```python
from build123d import *

# Parameters (mm, degrees)
SKETCH1_W           = 7
SKETCH1_H           = 7
BOSS_EXTRUDE1_DEPTH = 3
CUT_EXTRUDE1_DEPTH  = 7
CUT_EXTRUDE2_DEPTH  = 11
SKETCH4_R           = 1.8
CUT_EXTRUDE3_DEPTH  = 0.8
CUT_EXTRUDE4_DEPTH  = 0.4


with BuildPart() as part:
    # Sketch1 → Boss-Extrude1 (new body)
    with BuildSketch(Plane(origin=(0, 0, 0), x_dir=(1, 0, 0), z_dir=(0, 1, 0))):
        with Locations((3.5, 3.5)):
            Rectangle(SKETCH1_W, SKETCH1_H)
    extrude(amount=BOSS_EXTRUDE1_DEPTH)

    # Sketch2 → Cut-Extrude1 (cut)
    with BuildSketch(Plane.XY):
        Polygon((0, 0), (0.7, 3), (0, 3), align=None)
        Polygon((7, 0), (6.3, 3), (7, 3), align=None)
    extrude(amount=-CUT_EXTRUDE1_DEPTH, mode=Mode.SUBTRACT)

    # Sketch3 → Cut-Extrude2 (cut)
    with BuildSketch(Plane(origin=(0, 0, 0), x_dir=(0, 0, -1), z_dir=(1, 0, 0))):
        Polygon((0, 0), (0.7, 3), (0, 3), align=None)
        Polygon((7, 3), (6.3, 3), (7, 0), align=None)
    extrude(amount=CUT_EXTRUDE2_DEPTH, mode=Mode.SUBTRACT)

    # Sketch4 → Cut-Extrude3 (cut)
    with BuildSketch(Plane.XZ):
        with Locations(Location((3.5, -3.5, 0), (0, 0, 270))):
            Circle(SKETCH4_R)
    extrude(amount=-CUT_EXTRUDE3_DEPTH, mode=Mode.SUBTRACT)

    # Sketch5 → Cut-Extrude4 (cut)
    with BuildSketch(Plane(origin=(0, 3, 0), x_dir=(1, 0, 0), z_dir=(0, 1, 0))):
        with BuildLine():
            add(Edge.make_bspline(
                [(1.821714103, 3.488248698), (1.821961784, 3.531500253), (1.822448196, 3.616440725), (1.830876604, 3.741051587), (1.841985901, 3.86049575), (1.860077374, 3.974303397), (1.881359551, 4.083007187), (1.907977906, 4.186574853), (1.940043598, 4.284643186), (1.96555211, 4.347258757), (1.978064263, 4.377972255)],
                knots=[0, 0, 0, 0, 1.141009212, 2.240794809, 3.294380675, 4.305229195, 5.280013876, 6.216333343, 7.125095522, 8, 8, 8, 8], degree=3))
            add(Edge.make_bspline(
                [(1.978064263, 4.377972255), (1.998516886, 4.421635051), (2.039181575, 4.508447097), (2.114702293, 4.631119496), (2.200300575, 4.746809508), (2.295271713, 4.854910638), (2.397191064, 4.953795484), (2.506539435, 5.038426674), (2.619432008, 5.111662383), (2.699724257, 5.148495592), (2.739482532, 5.166734275)],
                knots=[0, 0, 0, 0, 1.031372299, 2.050613973, 3.077158538, 4.108712802, 5.127684358, 6.111366908, 7.06480644, 8, 8, 8, 8], degree=3))
            add(Edge.make_bspline(
                [(2.739482532, 5.166734275), (2.766470301, 5.177804055), (2.821019461, 5.200178904), (2.905795278, 5.228103887), (2.993787729, 5.250791674), (3.084360371, 5.271071912), (3.178392588, 5.285055803), (3.27512456, 5.296780816), (3.375085669, 5.302926099), (3.442700631, 5.303740345), (3.47706266, 5.304154146)],
                knots=[0, 0, 0, 0, 0.92659354, 1.872881803, 2.832850937, 3.813025581, 4.820167273, 5.851730198, 6.908245912, 8, 8, 8, 8], degree=3))
            add(Edge.make_bspline(
                [(3.47706266, 5.304154146), (3.538590536, 5.302611845), (3.659001433, 5.299593539), (3.834887941, 5.277792675), (4.001329981, 5.240979909), (4.157764144, 5.187771817), (4.305539157, 5.121260548), (4.443506895, 5.038760892), (4.571871554, 4.941165749), (4.690385205, 4.829813461), (4.797115236, 4.704898086), (4.890068226, 4.567586522), (4.968043218, 4.418522223), (5.032260126, 4.258116463), (5.081605981, 4.085845307), (5.117258315, 3.902194835), (5.138438688, 3.707029775), (5.140941529, 3.573137898), (5.142226923, 3.504374499)],
                knots=[0, 0, 0, 0, 1.064641025, 2.083517118, 3.061799897, 4.009540929, 4.938075217, 5.861300345, 6.78508344, 7.723570974, 8.670267188, 9.622657076, 10.586935816, 11.576069104, 12.607749008, 13.683335114, 14.81022093, 16, 16, 16, 16], degree=3))
            add(Edge.make_bspline(
                [(5.142226923, 3.504374499), (5.140971218, 3.436071549), (5.138526593, 3.303098467), (5.116950876, 3.109464875), (5.082776635, 2.92715322), (5.032236807, 2.75657997), (4.969936504, 2.596443536), (4.89115913, 2.448651271), (4.800152856, 2.311242808), (4.693574415, 2.187673494), (4.577055417, 2.075682155), (4.448853581, 1.979227653), (4.31189018, 1.896616215), (4.164920865, 1.829912739), (4.008903554, 1.777800449), (3.843329096, 1.740704804), (3.668112571, 1.718987832), (3.548170832, 1.715958568), (3.486878366, 1.714410557)],
                knots=[0, 0, 0, 0, 1.18845052, 2.313691126, 3.386664782, 4.412527756, 5.405809582, 6.372003093, 7.321919452, 8.268293321, 9.206237639, 10.129603466, 11.054616372, 11.9847576, 12.932764752, 13.912672021, 14.933336461, 16, 16, 16, 16], degree=3))
            add(Edge.make_bspline(
                [(3.486878366, 1.714410557), (3.424885779, 1.71596214), (3.303548476, 1.718999034), (3.126463104, 1.7406499), (2.959245037, 1.777757756), (2.802013351, 1.830053351), (2.653695695, 1.895743521), (2.51566143, 1.97751079), (2.387834254, 2.074576155), (2.270341671, 2.185249258), (2.163829132, 2.308455276), (2.072952075, 2.444980241), (1.994170592, 2.591328945), (1.931542745, 2.74971822), (1.881281222, 2.918518444), (1.847023473, 3.098700906), (1.825406036, 3.289769697), (1.822967241, 3.420879762), (1.821714103, 3.488248698)],
                knots=[0, 0, 0, 0, 1.080878253, 2.11558926, 3.1052859, 4.062802436, 5.000434901, 5.928596448, 6.853693179, 7.793554778, 8.738606028, 9.68692032, 10.647726704, 11.63151566, 12.651483354, 13.714466703, 14.825613081, 16, 16, 16, 16], degree=3))
        make_face()
        with BuildLine():
            add(Edge.make_bspline(
                [(2.494791026, 3.511385717), (2.495463421, 3.46297147), (2.496765502, 3.369218203), (2.510634389, 3.233137604), (2.531681539, 3.105921329), (2.562634465, 2.987713764), (2.601737596, 2.878429396), (2.649647038, 2.77797681), (2.7061648, 2.686206391), (2.772752717, 2.605055542), (2.844795621, 2.532603477), (2.92255951, 2.469914167), (3.004595136, 2.415957097), (3.092321967, 2.373358172), (3.183914249, 2.339551264), (3.280083591, 2.31448468), (3.381308169, 2.300720664), (3.450381011, 2.298746792), (3.485476122, 2.29774389)],
                knots=[0, 0, 0, 0, 1.313550922, 2.543666373, 3.708465049, 4.810029406, 5.85539231, 6.85404609, 7.825601258, 8.772642133, 9.696587791, 10.59409323, 11.479048685, 12.35559886, 13.234601248, 14.125357077, 15.047515647, 16, 16, 16, 16], degree=3))
            add(Edge.make_bspline(
                [(3.485476122, 2.29774389), (3.520575961, 2.298726471), (3.589658109, 2.30066035), (3.690758312, 2.31470579), (3.787118236, 2.338697967), (3.878346649, 2.372331634), (3.964859358, 2.415606978), (4.046581009, 2.468354444), (4.123040539, 2.531328963), (4.195005026, 2.602728481), (4.259795575, 2.684418325), (4.315832134, 2.776172907), (4.363717971, 2.877234741), (4.40282522, 2.987641635), (4.433016388, 3.107601318), (4.453204553, 3.23717726), (4.467185589, 3.375998963), (4.46848236, 3.471851744), (4.46915, 3.521201422)],
                knots=[0, 0, 0, 0, 0.949153107, 1.868086493, 2.754172764, 3.630100905, 4.492260106, 5.365378617, 6.254840125, 7.166615376, 8.102436631, 9.067266169, 10.06813181, 11.121736829, 12.23011542, 13.408501285, 14.665770308, 16, 16, 16, 16], degree=3))
            add(Edge.make_bspline(
                [(4.46915, 3.521201422), (4.468395892, 3.570074602), (4.466935489, 3.66472216), (4.45421689, 3.801791371), (4.433386174, 3.929313247), (4.404429177, 4.047254755), (4.366160687, 4.155634899), (4.320453453, 4.254750055), (4.265186916, 4.344082401), (4.20180297, 4.423585682), (4.131665715, 4.493563899), (4.055966759, 4.554826829), (3.974276008, 4.605801311), (3.88739075, 4.648689422), (3.794406419, 4.680507955), (3.696267954, 4.703716125), (3.592697629, 4.718007752), (3.521746781, 4.719869217), (3.485476122, 4.720820813)],
                knots=[0, 0, 0, 0, 1.332337092, 2.580197383, 3.749299508, 4.852775005, 5.886662144, 6.878700295, 7.822989687, 8.743523536, 9.644687758, 10.519443927, 11.392806431, 12.264866173, 13.155606721, 14.065961015, 15.011303331, 16, 16, 16, 16], degree=3))
            add(Edge.make_bspline(
                [(3.485476122, 4.720820813), (3.449200879, 4.719883854), (3.378241063, 4.718051022), (3.274509295, 4.703522778), (3.176061662, 4.681006152), (3.083090474, 4.647370777), (2.995448418, 4.604894527), (2.913459658, 4.552215512), (2.836478148, 4.49105655), (2.765712484, 4.420017304), (2.701301518, 4.339817822), (2.646008366, 4.249393926), (2.598858806, 4.149733156), (2.560175326, 4.040540508), (2.531498905, 3.9215156), (2.509458688, 3.79345835), (2.49708172, 3.655593683), (2.495571002, 3.560488178), (2.494791026, 3.511385717)],
                knots=[0, 0, 0, 0, 0.981996942, 1.920933313, 2.83127778, 3.712125466, 4.592427284, 5.463259035, 6.34592384, 7.249932058, 8.173122297, 9.125107726, 10.113123258, 11.154048744, 12.256187849, 13.424658091, 14.670364834, 16, 16, 16, 16], degree=3))
        make_face(mode=Mode.SUBTRACT)
    extrude(amount=-CUT_EXTRUDE4_DEPTH, mode=Mode.SUBTRACT)


solid = part.part
```
The model under review builds one solid part; all positions refer to its coordinate system, in mm. A direction names the side the tool comes from. Round coordinates to 2 decimals unless told otherwise and drop trailing zeros. Loops run counter-clockwise (first coordinate to the right, second up) from the corner with the lowest first, then second, coordinate; pieces in that order, holes last. Notation, with made-up numbers: (63, 30) -> (77, 30) arc R23 ccw to (77, 66) -> close; hole circle Ø6 at (66, -1.5). An arc over 180 degrees is marked (long way). Answer in a Markdown table with one row per item.
1) Draft analysis for pull direction Z (two halves, no side actions). For faces 1 (the flat face through (6.655, 1.479, -3.451)), 2 (the flat face through (4.6, 2.6, -3.9)), 3 (the flat face through (3.451, 1.479, -0.345)), state which applies: pulls with the +Z half, pulls with the -Z half, needs draft (parallel to the pull), parting line crosses it, or undercut.
Taken from the geometry:
| item | result |
|---|---|
| face 1 | needs draft |
| face 2 | undercut |
| face 3 | pulls with the +Z half |
2) Wall thickness on line 1 along Z through (x, y) = (4.25, 2.7); line 2 along X through (y, z) = (0.3, -3.5); line 3 along Z through (x, y) = (3.25, 0.2): over which ranges is each line inside the solid? List them lowest first.
Taken from the geometry:
| item | result |
|---|---|
| line 1 | z = -6.37 to -5.15, -4.36 to -2.67, -1.87 to -0.63 |
| line 2 | x = 0.07 to 1.7, 5.3 to 6.93 |
| line 3 | z = -6.95 to -5.28, -1.72 to -0.05 |
3) Tool access review of faces 4 (the flat face through (4, 0.8, -3)), 5 (the flat face through (3.451, 1.521, -6.645)): name each direction out of +Z, -Z, +X, -X, +Y, -Y from which nothing blocks a thin tool from reaching the whole face with its end or side.
Taken from the geometry:
| item | result |
|---|---|
| face 4 | -Y |
| face 5 | -Z, +X, -X, +Y |
4) Consider section A-A, the plane x = 1. Write out the cut boundary in (y, z).
Taken from the geometry:
| item | result |
|---|---|
| outline | (0, -7) -> (3, -6.3) -> (3, -0.7) -> (0, 0) -> close |
5) Consider section B-B, the plane z = -1.25. Write out the cut boundary in (x, y).
Taken from the geometry:
| item | result |
|---|---|
| outline | (0, 0) -> (7, 0) -> (6.3, 3) -> (0.7, 3) -> close |
6) For pin 1 Ø1.8 at (x, z) = (4, -4) entering from -Y, flat-tipped, find the tip position at first contact; note if it passes through.
Taken from the geometry:
| item | result |
|---|---|
| pin 1 | stops at y = 0.8 |
